Autodesk Inventor part; units mm, degrees
ref_plane "Work Plane2" through (2.032, 0, 0) normal (0, 1, 0) x (1, 0, 0)
ref_plane "YZ Plane" through (0, 0, 0) normal (1, 0, 0) x (0, 1, 0)
ref_plane "XZ Plane" through (0, 0, 0) normal (0, 1, 0) x (-1, 0, 0)
sketch "Sketch1" plane through (0, 0, 0) normal (0, 0, 1) x (1, 0, 0)
  line L0 (2.1844, 0) -> (50.8, 0)
  line L1 (50.8, 0) -> (50.8, 1.7526)
  line L2 (50.8, 1.7526) -> (1.524, 1.7526)
  line L3 (0.4583, 3.0226) -> (0, 3.0226)
  line L4 (-5.08, 0) -> (30.48, 0)
  line L5 (0, -0.6045) -> (0, 3.6271)
  line L6 (0, 1.9558) -> (1.5573, 1.1793)
  line L7 (1.5573, 1.1793) -> (2.1844, 0)
  line L8 (1.524, 1.7526) -> (0.4583, 3.0226)
  line L9 (0, 3.0226) -> (0, 1.9558)
  dimension "d2" = 3.5052
  dimension "d3" = 6.0452
  dimension "d4" = 2.1844
  dimension "d5" = 3.9116
  dimension "d6" = 26.5
  dimension "d7" = 62
  dimension "d13" = 50
  dimension "d14" = 1.524
  dimension "d15" = 50.8
revolve "Body" add sketch "Sketch1" angle 360 about axis through (2.1844, 0, 0) along (1, 0, 0) contours L7 L6 L5 L3 L8 L2 L1 L0
sketch "Sketch2" plane through (0, 0, 0) normal (-1, 0, 0) x (0, 0, 1)
  line L0 (0, -4.2316) -> (0, 4.2316)
  line L1 (-4.2316, 0) -> (4.2316, 0)
  line L2 (0, 1.9558) -> (0, 0) construction
  line L3 (0, 0) -> (1.9558, 0) construction
  arc A0 (0.6519, 0) -> (0, 0.6519) centre (0, 0) ccw
  line L4 (0, 0) -> (0.7947, 0.7947) construction
  arc A1 (0.9779, 0) -> (0, 0.9779) centre (0, 0) ccw construction
  line L5 (0.3429, 1.9255) -> (0.2811, 0.9366)
  line L6 (1.9255, 0.3429) -> (0.9366, 0.2811)
  arc A2 (0.2811, 0.9366) -> (0.9366, 0.2811) centre (0.8981, 0.8981) ccw
  arc A3 (1.9558, 0) -> (1.9255, 0.3429) centre (0, 0) ccw
  arc A4 (0.3429, 1.9255) -> (0, 1.9558) centre (0, 0) ccw
  arc A5 (1.9255, 0.3429) -> (0.3429, 1.9255) centre (0, 0) ccw
  line L7 (0.3429, -1.9255) -> (0.2811, -0.9366)
  line L8 (1.9255, -0.3429) -> (0.9366, -0.2811)
  arc A6 (0.9366, -0.2811) -> (0.2811, -0.9366) centre (0.8981, -0.8981) ccw
  arc A7 (1.9255, -0.3429) -> (1.9558, 0) centre (0, 0) ccw
  arc A8 (0, -1.9558) -> (0.3429, -1.9255) centre (0, 0) ccw
  arc A9 (0.3429, -1.9255) -> (1.9255, -0.3429) centre (0, 0) ccw
  line L9 (-0.3429, 1.9255) -> (-0.2811, 0.9366)
  line L10 (-1.9255, 0.3429) -> (-0.9366, 0.2811)
  arc A10 (-0.9366, 0.2811) -> (-0.2811, 0.9366) centre (-0.8981, 0.8981) ccw
  arc A11 (-1.9255, 0.3429) -> (-1.9558, 0) centre (0, 0) ccw
  arc A12 (0, 1.9558) -> (-0.3429, 1.9255) centre (0, 0) ccw
  arc A13 (-0.3429, 1.9255) -> (-1.9255, 0.3429) centre (0, 0) ccw
  arc A14 (-1.9255, -0.3429) -> (-0.3429, -1.9255) centre (0, 0) ccw
  arc A15 (-0.3429, -1.9255) -> (0, -1.9558) centre (0, 0) ccw
  arc A16 (-1.9558, 0) -> (-1.9255, -0.3429) centre (0, 0) ccw
  line L11 (-1.9255, -0.3429) -> (-0.9366, -0.2811)
  arc A17 (-0.2811, -0.9366) -> (-0.9366, -0.2811) centre (-0.8981, -0.8981) ccw
  line L12 (-0.3429, -1.9255) -> (-0.2811, -0.9366)
  dimension "d18" = 45
  dimension "d19" = 1.3039
  dimension "d20" = 1.9558
  dimension "d21" = 3.9116
  dimension "d22" = 0.3429
extrude "Slot" add sketch "Sketch2" against normal up to next contours A2 L5 A5 L6 | L9 A10 L10 A13 | L7 A6 L8 A9 | A14 L11 A17 L12
fillet "Fillet1" radius 0.1372 4 edges at (0, 1.9558, 0) (0, 0, 1.9558) (0, -1.9558, 0) (0, 0, -1.9558)
thread "Thread"
chamfer "Chamfer1" distance 0.4723 distance2 0.4723 1 edges at (50.8, -1.7526, 0) measured on face at (50.8, -0.4673, -0.1398)
ref_plane "Work Plane2" through (2.032, 0, 0) normal (0, 1, 0) x (1, 0, 0)
equation "\"d2\" = GD"
equation "\"d3\" = KOD"
equation "\"d4\" = INTI"
equation "\"d5\" = SDM"
equation "\"d13\" = 0.5 * SEWI"
equation "\"d14\" = KOH"
equation "\"d19\" = 0.333333 * SDM"
equation "\"d20\" = 0.5 * SDM"
equation "\"d21\" = SDM"
equation "\"d22\" = 0.5 * SBR"
equation "\"d45\" = INTI"
equation "\"d25\" = 0.2 * SBR"
equation "\"d9\" = GEL"
equation "\"d11\" = -0.5 * SPD + 0.5 * GD"
equation "\"d12\" = GUL"
equation "\"GD\" = NND"
equation "\"NLG\" = 25.4"
equation "\"GEL\" = 19.05"
equation "\"KOD\" = 6.0452"
equation "\"KOH\" = 1.524"
equation "\"SDM\" = 3.9116"
equation "\"INTI\" = 2.1844"
equation "\"SBR\" = 0.6858"
equation "\"GUL\" = -0.5 * SPD + 0.5 * NND"
equation "\"SPD\" = 2.56064"
equation "\"SEWI\" = 100deg"
equation "\"d1\" = KOH"
equation "\"d17\" = SDM"
equation "\"TOA\" = 30deg"
equation "\"EPV\" = 2.99461"
equation "\"THREADDIA\" = 3.5052"
equation "\"BDM\" = NND"
equation "\"NND\" = 3.5052"
equation "\"GAL\" = 0.79375"
equation "\"GD1\" = SPD"
properties part number "ANSI B18.6.3 - 6-32 UNC x 1, CRFCHMSTII(2)" material "Steel, Mild"
Geometry: final body of the model. Coordinates: model frame, mm. A direction names the side the tool comes from. Give positions to 0.01 mm unless a question says otherwise; leave off trailing zeros. Loops run counter-clockwise (first coordinate to the right, second up) from the corner with the lowest first, then second, coordinate; pieces in that order, holes last. Notation, with made-up numbers: (73, -11) -> (84, -11) arc R20 ccw to (84, 6) -> close; hole circle Ø8 at (65.25, -39). An arc over 180 degrees is marked (long way). Return JSON: item names as keys, results as strings.
Item 1: Mould query, pull axis Y, two halves, no side actions, for faces 4 (the flat face through (50.8, 0, 0)), 5 (the flat face through (0.64, 1.24, -0.3)), 6 (the cylindrical face through (0.23, -0.66, 2.95)). Classes: released by +Y, released by -Y, zero draft, split by the parting line, or undercut.
Filled in:
{"face 4": "zero draft", "face 5": "undercut", "face 6": "split by the parting line"}
Item 2: Section A-A, the plane x = 20.5. Output: boundary loops of the cut face in (y, z), plus the area to 3 significant figures.
Filled in:
{"outline": "circle Ø3.51 at (0, 0)", "area": "9.65 mm^2"}
Item 3: Line query: line 1 (X direction, y = 1.25, z = 1.75); line 2 (X direction, y = -1.75, z = -0.75); line 3 (Z direction, x = 31, y = 1.5). Output: solid intervals per line, ascending.
Filled in:
{"line 1": "0 to 1.19", "line 2": "0 to 1.4", "line 3": "-0.91 to 0.91"}
Item 4: Access query for faces 1 (the flat face through (0.64, -0.3, -1.24)), 2 (the flat face through (0, 1, -1)), 3 (the cylindrical face through (25.58, 1.67, -0.53)). Directions: +Z, -Z, +X, -X, +Y, -Y. A direction counts if a zero-diameter tool reaches every point of the face in a straight line with its end or side. Return the directions, or none.
Filled in:
{"face 1": "-X", "face 2": "+Z, -Z, -X, +Y, -Y", "face 3": "+X"}
Item 5: Pin query (flat end, axial travel): P1, Ø1.5, axis at x = 31.5, y = 2, coming from the -Z side; P2, Ø1, axis at x = 40, y = -2, coming from the -Z side; P3, Ø1.5, axis at x = 19.5, y = 0.5, coming from the -Z side. Return the tip coordinate at first contact, or that it passes through.
Filled in:
{"P1": "z = -1.23", "P2": "z = -0.91", "P3": "z = -1.75"}
